from build123d import *

# Parameters (mm, degrees)
F0_W     = 222.1541649566
F0_H     = 100
F0_W_2   = 395.4195475671
F0_W_3   = 188.4643873005
F0_W_4   = 100
F0_H_2   = 361.5790828629
F0_H_3   = 156.8592581168
F0_H_4   = 152.8593497919
F0_W_5   = 170.2914773738
F0_W_6   = 779.0951247443
F0_H_5   = 292.5978301498
F1_DEPTH = 500
F2_W     = 1910.4056636256
F2_H     = 1200
F3_DEPTH = 100
F5_DEPTH = 1200


with BuildPart() as f1:
    # F0 (on Top) → F1 (new body)
    with BuildSketch(Plane.XY):
        Polygon((-1039.4755020642, -481.5616590203), (-939.4755020642, -481.5616590203), (-939.4755020642, 0), (-939.4755020642, 100), (-939.4755020642, 518.4383409797), (-1039.4755020642, 518.4383409797), align=None)
        Polygon((-710.1491273506, -481.5616590203), (-939.4755020642, -481.5616590203), (-1039.4755020642, -481.5616590203), (-1039.4755020642, -581.5616590203), (-710.1491273506, -581.5616590203), align=None)
        Polygon((-1039.4755020642, 618.4383409797), (-1039.4755020642, 518.4383409797), (-939.4755020642, 518.4383409797), (-659.1245005101, 518.4383409797), (-659.1245005101, 618.4383409797), align=None)
        with Locations((-548.0474180319, 568.4383409797)):
            Rectangle(F0_W, F0_H)
        Polygon((-436.9703355536, 618.4383409797), (-436.9703355536, 518.4383409797), (-160.3803773199, 518.4383409797), (-60.3803773199, 518.4383409797), (-60.3803773199, 618.4383409797), (-81.4295849381, 618.4383409797), align=None)
        with Locations((137.3293964637, 568.4383409797)):
            Rectangle(F0_W_2, F0_H)
        with Locations((429.2713638974, 568.4383409797)):
            Rectangle(F0_W_3, F0_H)
        Polygon((523.5035575476, 618.4383409797), (523.5035575476, 518.4383409797), (770.9301615614, 518.4383409797), (870.9301615614, 518.4383409797), (870.9301615614, 618.4383409797), align=None)
        with Locations((820.9301615614, 337.6487995483)):
            Rectangle(F0_W_4, F0_H_2)
        with Locations((820.9301615614, 78.4296290584)):
            Rectangle(F0_W_4, F0_H_3)
        with Locations((820.9301615614, -76.429674896)):
            Rectangle(F0_W_4, F0_H_4)
        Polygon((770.9301615614, -481.5616590203), (770.9301615614, -581.5616590203), (870.9301615614, -581.5616590203), (870.9301615614, -170.4701158022), (870.9301615614, -152.8593497919), (770.9301615614, -152.8593497919), align=None)
        Polygon((439.6196226801, -499.1724250305), (439.6196226801, -581.5616590203), (770.9301615614, -581.5616590203), (770.9301615614, -481.5616590203), (539.6196226801, -481.5616590203), (539.6196226801, -236.3492257267), (439.6196226801, -236.3492257267), (439.6196226801, -481.5616590203), align=None)
        Polygon((-160.3803773199, -258.3257411009), (-160.3803773199, -481.5616590203), (-160.3803773199, -508.6633241055), (-160.3803773199, -581.5616590203), (-60.3803773199, -581.5616590203), (-60.3803773199, -258.3257411009), align=None)
        with Locations((-625.0033886637, -531.5616590203)):
            Rectangle(F0_W_5, F0_H)
        with Locations((-549.927939692, 50)):
            Rectangle(F0_W_6, F0_H)
        Polygon((-160.3803773199, -481.5616590203), (-539.8576499768, -481.5616590203), (-539.8576499768, -581.5616590203), (-160.3803773199, -581.5616590203), (-160.3803773199, -508.6633241055), align=None)
        Polygon((-160.3803773199, 100), (-160.3803773199, 0), (-160.3803773199, -145.845679975), (-60.3803773199, -145.845679975), (-60.3803773199, 100), align=None)
        with Locations((-110.3803773199, 372.1394259048)):
            Rectangle(F0_W_4, F0_H_5)
    extrude(amount=F1_DEPTH)

    # F2 (on face) → F3 (join)
    with BuildSketch(Plane.XY.offset(500)):
        with Locations((-84.2726702514, 18.4383409797)):
            Rectangle(F2_W, F2_H)
    extrude(amount=F3_DEPTH)

    # F4 (on face) → F5 (join)
    with BuildSketch(Plane.XZ.offset(581.5616590203)):
        Polygon((-1039.4755020642, 1188.9448165894), (-1039.4755020642, 600), (870.9301615614, 600), (1038.4503075273, 544.0466226834), (1057.0495128632, 592.2645926476), (-1211.7080801369, 1467.3965893042), (-1231.8549156189, 1435.4420900345), (-1039.4755020642, 1314.1497373581), align=None)
    extrude(amount=-F5_DEPTH)


solid = f1.part
For this review, take the finished solid that the model builds, in its own axes (mm). A direction names the side the tool comes from. Give positions to 0.01 mm unless a question says otherwise; leave off trailing zeros. Loops run counter-clockwise (first coordinate to the right, second up) from the corner with the lowest first, then second, coordinate; pieces in that order, holes last. Notation, with made-up numbers: (60.25, 29) -> (102.25, 29) arc R10 cw to (102.25, 33) -> close; hole circle Ø4 at (22, 41.5). An arc over 180 degrees is marked (long way). One line per question, with ' | ' between items.
1) Insertion check: pin 1 Ø2 at (x, y) = (-12.5, 41.5) entering from -Z; pin 2 Ø4 at (y, z) = (-192.5, 259.5) entering from -X; pin 3 Ø6 at (x, y) = (-741, -292) entering from +Z. Each pin has a flat end and moves straight along its axis. Give the tip position at first contact, or say it passes through.
Resolved:
pin 1: stops at z = 500 | pin 2: stops at x = -1039.48 | pin 3: stops at z = 1286.99
2) To check wall thickness, follow probe 1 along Y at (x, z) = (-764, 89); probe 2 along X at (y, z) = (406, 424); probe 3 along X at (y, z) = (214.5, 162). State the ranges of each line that lie inside material, in increasing order.
Resolved:
probe 1: y = -581.56 to -481.56, 0 to 100, 518.44 to 618.44 | probe 2: x = -1039.48 to -939.48, -160.38 to -60.38, 770.93 to 870.93 | probe 3: x = -1039.48 to -939.48, 770.93 to 870.93
3) We need section D-D (y = 142.5). Write out the cut boundary in (x, z).
Resolved:
outline: (-1231.85, 1435.44) -> (-1039.48, 1314.15) -> (-1039.48, 0) -> (-939.48, 0) -> (-939.48, 500) -> (770.93, 500) -> (770.93, 0) -> (870.93, 0) -> (870.93, 600) -> (1038.45, 544.05) -> (1057.05, 592.26) -> (-1211.71, 1467.4) -> close
4) We need section C-C (x = -558.5). Write out the cut boundary in (y, z).
Resolved:
outline: (-581.56, 0) -> (-481.56, 0) -> (-481.56, 500) -> (0, 500) -> (0, 0) -> (100, 0) -> (100, 500) -> (518.44, 500) -> (518.44, 0) -> (618.44, 0) -> (618.44, 1215.43) -> (-581.56, 1215.43) -> close
5) We need section A-A (z = 151.5). Write out the cut boundary in (x, y), plus the area to 3 significant figures.
Resolved:
outline: (-1039.48, -581.56) -> (-60.38, -581.56) -> (-60.38, -258.33) -> (-160.38, -258.33) -> (-160.38, -481.56) -> (-939.48, -481.56) -> (-939.48, 0) -> (-160.38, 0) -> (-160.38, -145.85) -> (-60.38, -145.85) -> (-60.38, 100) -> (-939.48, 100) -> (-939.48, 518.44) -> (-160.38, 518.44) -> (-160.38, 225.84) -> (-60.38, 225.84) -> (-60.38, 518.44) -> (770.93, 518.44) -> (770.93, -481.56) -> (539.62, -481.56) -> (539.62, -236.35) -> (439.62, -236.35) -> (439.62, -581.56) -> (870.93, -581.56) -> (870.93, 618.44) -> (-1039.48, 618.44) -> close | area: 711,000 mm2
6) For faces 3 (the flat face through (439.62, -407, 246)), 4 (the flat face through (-103, 618.438, 581)), 5 (the flat face through (-494, 100, 246)), list the 3-axis set-ups (+Z, -Z, +X, -X, +Y, -Y) from which the entire face can be reached by the end or side of a thin tool; tool diameter is ignored.
Resolved:
face 3: -Z, -Y | face 4: +Z, -Z, +X, -X, +Y | face 5: -Z
7) The part is to be moulded in two halves that separate along X. For faces 1 (the flat face through (-358, -581.562, 581)), 2 (the flat face through (-60.38, -25, 246)), say which applies: +X half, -X half, draft (parallel to the pull), parting line (faces both ways), or undercut.
Resolved:
face 1: draft | face 2: undercut
8) We need section B-B (y = 339). Write out the cut boundary in (x, z), plus the area to 3 significant figures.
Resolved:
outline: (-1231.85, 1435.44) -> (-1039.48, 1314.15) -> (-1039.48, 0) -> (-939.48, 0) -> (-939.48, 500) -> (-160.38, 500) -> (-160.38, 0) -> (-60.38, 0) -> (-60.38, 500) -> (770.93, 500) -> (770.93, 0) -> (870.93, 0) -> (870.93, 600) -> (1038.45, 544.05) -> (1057.05, 592.26) -> (-1211.71, 1467.4) -> close | area: 1,190,000 mm2
